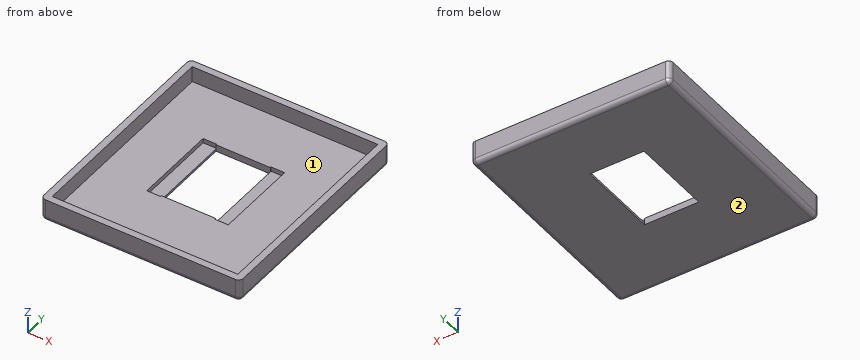
Autodesk Inventor part; units mm, degrees
ref_plane "YZ Plane" through (0, 0, 0) normal (1, 0, 0) x (0, 1, 0)
ref_plane "XZ Plane" through (0, 0, 0) normal (0, 1, 0) x (-1, 0, 0)
ref_plane "XY Plane" through (0, 0, 0) normal (0, 0, 1) x (1, 0, 0)
sketch "Esquisse8" plane through (0, 0, 0) normal (0, 0, 1) x (1, 0, 0)
  line L0 (3, 3) -> (85, 3)
  line L1 (85, 3) -> (85, 95)
  line L2 (85, 95) -> (3, 95)
  line L3 (3, 95) -> (3, 3)
  line L4 (0, 0) -> (88, 0)
  line L5 (88, 0) -> (88, 98)
  line L6 (88, 98) -> (0, 98)
  line L7 (0, 98) -> (0, 0)
  dimension "d34" = 3
  dimension "d35" = 3
  dimension "d36" = 3
  dimension "d37" = 92
  dimension "d38" = 88
  dimension "d39" = 3
  dimension "d51" = 92
extrude "Extrusion5" add sketch "Esquisse8" along normal blind 10 contours L3 L2 L1 L0 | L7 L6 L5 L4
shell "Coque5" thickness 3 removed faces 1 at (58.6667, 32.6667, 10)
sketch "Esquisse9" plane through (3, 3, 3) normal (0, 0, 1) x (1, 0, 0)
  line L0 (52, 66) -> (64, 66)
  line L1 (64, 66) -> (64, 30)
  line L2 (64, 30) -> (52, 30)
  line L3 (52, 30) -> (52, 66)
  line L4 (82, 92) -> (82, 0)
  line L5 (0, 0) -> (82, 0)
  line L6 (0, 92) -> (0, 0)
  line L7 (52, 30) -> (28, 30)
  line L8 (28, 30) -> (28, 66)
  line L9 (28, 66) -> (52, 66)
  line L10 (52, 66) -> (52, 30)
  point P0 (-3, -3)
  dimension "d49" = 18
  dimension "d52" = 30
  dimension "d53" = 52
  dimension "d56" = 36
  dimension "d59" = 24
  dimension "d60" = 36
extrude "Extrusion6" cut sketch "Esquisse9" against normal blind 3 contours L3 L7 L8 L9
sketch "Esquisse11" plane through (3, 3, 3) normal (0, 0, 1) x (1, 0, 0)
  point P0 (-3, -3)
sketch "Esquisse12" plane through (3, 3, 3) normal (0, 0, 1) x (1, 0, 0)
  line L0 (28, 66.4268) -> (22, 66.4268)
  line L1 (22, 66.4268) -> (22, 29.4268)
  line L2 (22, 29.4268) -> (28, 29.4268)
  line L3 (28, 29.4268) -> (28, 66.4268)
  line L4 (28, 30) -> (28, 66)
  point P0 (-3, -3)
  dimension "d63" = 6
  dimension "d64" = 37
extrude "Extrusion7" cut sketch "Esquisse12" along normal mid plane 4
ref_plane "Plan de construction2" through (44, 3, 3) normal (1, 0, 0) x (0, 0, -1)
sketch "Esquisse13" plane through (3, 3, 3) normal (0, 0, 1) x (1, 0, 0)
  line L0 (52, 66.4584) -> (58, 66.4584)
  line L1 (58, 66.4584) -> (58, 29.4584)
  line L2 (58, 29.4584) -> (52, 29.4584)
  line L3 (52, 29.4584) -> (52, 66.4584)
  line L4 (52, 66) -> (52, 30)
  point P0 (-3, -3)
  dimension "d67" = 6
  dimension "d68" = 37
extrude "Extrusion8" cut sketch "Esquisse13" along normal mid plane 4
fillet "Congé2" radius 2 8 edges at (0, 0, 5) (0, 98, 5) (44, 98, 0) (88, 98, 5) (88, 0, 5) (88, 49, 0) (0, 49, 0) (44, 0, 0)
properties part number "couvercle 2" material "Plastique ABS"
The model under review builds one solid part; all positions refer to its coordinate system, in mm. Face numbers are marked on the shaded views. Round coordinates to 2 decimals unless told otherwise and drop trailing zeros. Loops run counter-clockwise (first coordinate to the right, second up) from the corner with the lowest first, then second, coordinate; pieces in that order, holes last. Notation, with made-up numbers: (21.5, 62) -> (25.5, 62) arc R12 cw to (25.5, 85) -> close; hole circle Ø4 at (16.25, -32.5). An arc over 180 degrees is marked (long way). Answer as a JSON object with one key per item and string values. Group by question number.
1) We need section C-C on y = 80.5. Write out the cut boundary in (x, z).
2) Mouldability with a two-part tool opening along Y and no side actions: class the marked faces 1 and 2 as released by +Y, released by -Y, zero draft, split by the parting line, or undercut.
3) For pin 1 Ø1.1 at (y, z) = (48.5, 0.5) entering from +X; pin 2 Ø0.6 at (y, z) = (32.5, 1.5) entering from -X; pin 3 Ø6.5 at (x, y) = (28.5, 60) entering from +Z, all flat-tipped, find the tip position at first contact; note any pin that passes through.
4) We need section B-B on z = 4.25. Write out the cut boundary in (x, y).
5) We need section A-A on x = 34.5. Write out the cut boundary in (y, z), then the cut area to 3 significant figures.
6) For line 1 (X direction, y = 66, z = 5.25); line 2 (Y direction, x = 21, z = 5); line 3 (Y direction, x = 38, z = 2.75), list the stretches that pass through material, from the lowest coordinate up. Write a range as [from, to].
7) We need section D-D on x = 12.5. Write out the cut boundary in (y, z).
Result set:
{
 "1": {"outline": "(0, 2) arc R2 ccw to (2, 0) -> (86, 0) arc R2 ccw to (88, 2) -> (88, 10) -> (85, 10) -> (85, 3) -> (3, 3) -> (3, 10) -> (0, 10) -> close"},
 "2": {"face 1": "undercut", "face 2": "zero draft"},
 "3": {"pin 1": "x = 87.76", "pin 2": "x = 0.01", "pin 3": "z = 1"},
 "4": {"outline": "(0, 2) arc R2 ccw to (2, 0) -> (86, 0) arc R2 ccw to (88, 2) -> (88, 96) arc R2 ccw to (86, 98) -> (2, 98) arc R2 ccw to (0, 96) -> close; hole (3, 3) -> (85, 3) -> (85, 95) -> (3, 95) -> close"},
 "5": {"outline": "(0, 2) arc R2 ccw to (2, 0) -> (33, 0) -> (33, 3) -> (3, 3) -> (3, 10) -> (0, 10) -> close; (69, 0) -> (96, 0) arc R2 ccw to (98, 2) -> (98, 10) -> (95, 10) -> (95, 3) -> (69, 3) -> close", "area": "226 mm²"},
 "6": {"line 1": "[0, 3], [85, 88]", "line 2": "[0, 3], [95, 98]", "line 3": "[0, 33], [69, 98]"},
 "7": {"outline": "(0, 2) arc R2 ccw to (2, 0) -> (96, 0) arc R2 ccw to (98, 2) -> (98, 10) -> (95, 10) -> (95, 3) -> (3, 3) -> (3, 10) -> (0, 10) -> close"}
}
